The model under review builds one solid part; all positions refer to its coordinate system, in mm. Face numbers are marked on the shaded views. A direction names the side the tool comes from. Round coordinates to 2 decimals unless told otherwise and drop trailing zeros. Loops run counter-clockwise (first coordinate to the right, second up) from the corner with the lowest first, then second, coordinate; pieces in that order, holes last. Notation, with made-up numbers: (15.25, 60.25) - (73.25, 60.25) arc R13 ccw to (73.25, 81.25) - close; hole circle Ø3 at (62.25, 33). An arc over 180 degrees is marked (long way). Answer as CSV lines item,"result".
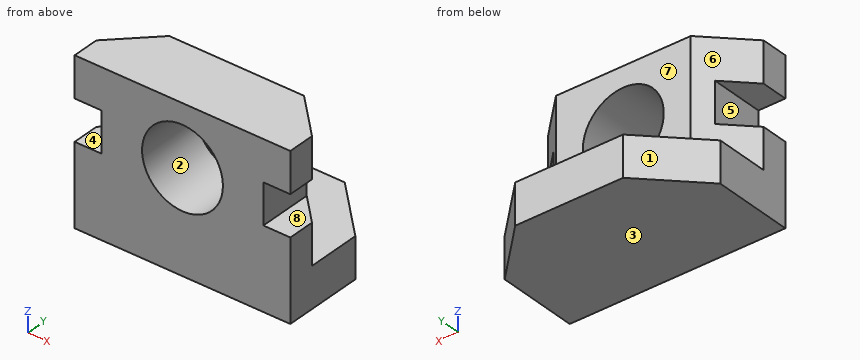
Autodesk Inventor part; units mm, degrees
ref_plane "YZ Plane" through (0, 0, 0) normal (1, 0, 0) x (0, 1, 0)
ref_plane "XZ Plane" through (0, 0, 0) normal (0, 1, 0) x (-1, 0, 0)
ref_plane "XY Plane" through (0, 0, 0) normal (0, 0, 1) x (1, 0, 0)
sketch "草圖1" plane through (0, 0, 0) normal (0, 0, 1) x (1, 0, 0)
  line L0 (0, 0) -> (0, 8)
  line L1 (0, 8) -> (12, 20)
  line L2 (12, 20) -> (52, 20)
  line L3 (52, 20) -> (64, 8)
  line L4 (64, 8) -> (64, 0)
  line L5 (64, 0) -> (0, 0)
  dimension "d0" = 8
  dimension "d1" = 8
  dimension "d2" = 40
  dimension "d3" = 64
  dimension "d4" = 20
  dimension "d5" = 12
extrude "擠出1" add sketch "草圖1" against normal blind 36
sketch "草圖3" plane through (12, 20, 0) normal (0, 1, 0) x (1, 0, 0)
  line L0 (52, 0) -> (52, 36)
  line L1 (52, 24) -> (44, 24)
  line L2 (44, 24) -> (44, 12)
  line L3 (44, 12) -> (52, 12)
  line L4 (40, 0) -> (52, 0)
  point P0 (-12, 0)
  dimension "d10" = 12
  dimension "d11" = 12
  dimension "d12" = 8
extrude "擠出2" cut sketch "草圖3" against normal blind 48
sketch "草圖5" plane through (12, 20, 0) normal (0, 1, 0) x (1, 0, 0)
  line L0 (-12, 0) -> (-12, 36)
  line L1 (-12, 12) -> (-4, 12)
  line L2 (-4, 12) -> (-4, 24)
  line L3 (-4, 24) -> (-12, 24)
  line L4 (-12, 0) -> (0, 0)
  dimension "d18" = 12
  dimension "d19" = 12
  dimension "d20" = 8
extrude "擠出3" cut sketch "草圖5" against normal blind 48
sketch "草圖6" plane through (12, 20, 0) normal (0, 1, 0) x (1, 0, 0)
  circle A0 centre (20, 18) radius 12
  line L0 (0, 0) -> (40, 0)
  line L1 (40, 0) -> (40, 36)
  point P0 (-12, 0)
  dimension "d23" = 24
  dimension "d24" = 18
  dimension "d25" = 20
extrude "擠出4" cut sketch "草圖6" against normal blind 48
sketch "草圖7" plane through (0, 0, -36) normal (0, 0, -1) x (-1, 0, 0)
  line L0 (-64, 0) -> (-64, 24)
  line L1 (-64, 24) -> (-48, 40)
  line L2 (-48, 40) -> (-16, 40)
  line L3 (-16, 40) -> (0, 24)
  line L4 (0, 0) -> (0, 8)
  line L5 (0, 24) -> (0, 8)
  line L6 (0, 8) -> (0, 0)
  line L7 (-64, 0) -> (0, 0)
  dimension "d28" = 32
  dimension "d29" = 16
  dimension "d30" = 40
  dimension "d31" = 16
  dimension "d32" = 16
extrude "擠出5" add sketch "草圖7" along normal blind 12
properties part number "410571040加分題"
1. Take a section at A-A (y = 17.5). State the section outline as (x, z) points.
Numbers:
outline,"(0, -48) - (64, -48) - (64, -36) - (54.5, -36) - (54.5, 0) - (9.5, 0) - (9.5, -36) - (0, -36) - close; hole circle Ø24 at (32, -18)"
2. Clearance check with flat-ended pins moving along their axes: pin 1 (19 mm diameter, centred on x = 32, z = -18, fed in from +Y); pin 2 (6 mm diameter, centred on y = 10.5, z = -20.5, fed in from -X); pin 3 (1.5 mm diameter, centred on x = 51.5, z = -24.5, fed in from +Y); pin 4 (9.5 mm diameter, centred on x = 35, y = 21, fed in from +Z). State where each tip first meets the part, or that it passes through.
Numbers:
pin 1,"passes through"
pin 2,"stops at x = 8"
pin 3,"stops at y = 20"
pin 4,"stops at z = 0"
3. Wall thickness on probe 1 along Z at (x, y) = (32, 5.5); probe 2 along X at (y, z) = (14, -18); probe 3 along Z at (x, y) = (54, 23.5): over which ranges is each line inside the solid? List them lowest first.
Numbers:
probe 1,"z = -48 to -30, -6 to 0"
probe 2,"x = 8 to 20, 44 to 56"
probe 3,"z = -48 to -36"
4. Take a section at C-C (x = 32). State the section outline as (y, z) points.
Numbers:
outline,"(0, -48) - (40, -48) - (40, -36) - (20, -36) - (20, -30) - (0, -30) - close; (0, -6) - (20, -6) - (20, 0) - (0, 0) - close"
5. Take a section at B-B (z = -18). State the section outline as (x, y) points, plus the area to 3 significant figures.
Numbers:
outline,"(8, 0) - (20, 0) - (20, 20) - (12, 20) - (8, 16) - close; (44, 0) - (56, 0) - (56, 16) - (52, 20) - (44, 20) - close"
area,"464 mm²"
6. Tool access review of the marked faces 5, 6, 7 and 8: name each direction out of +Z, -Z, +X, -X, +Y, -Y from which nothing blocks a thin tool from reaching the whole face with its end or side.
Numbers:
face 5,"-X, +Y, -Y"
face 6,"+Z, -X, +Y"
face 7,"+Z, +X, -X, +Y"
face 8,"+X, +Y, -Y"
7. Draft analysis for pull direction Z (two halves, no side actions). For the marked faces 1, 2, 3 and 4, state which applies: +Z half, -Z half, draft (parallel to the pull), parting line (faces both ways), or undercut.
Numbers:
face 1,"draft"
face 2,"undercut"
face 3,"-Z half"
face 4,"undercut"
8. Take a section at D-D (z = -41). State the section outline as (x, y) points, plus the area to 3 significant figures.
Numbers:
outline,"(0, 0) - (64, 0) - (64, 24) - (48, 40) - (16, 40) - (0, 24) - close"
area,"2,300 mm²"
